```python
from build123d import *

# Parameters (mm, degrees)
F0_R          = 12.5
F1_DEPTH      = 20
F2_R          = 15
F3_DEPTH      = 4
F5_DEPTH      = 12
F7_DEPTH      = 7.4
F7_DEPTH_BACK = 5.4
F8_SIZE       = 0.5


with BuildPart() as f1:
    # F0 (on Top) → F1 (new body)
    with BuildSketch(Plane.XY):
        Circle(F0_R)
    extrude(amount=F1_DEPTH)

    # F2 (on face) → F3 (join)
    with BuildSketch(Plane.XY.offset(20)):
        Circle(F2_R)
    extrude(amount=F3_DEPTH)

    # F4 (on face) → F5 (join)
    with BuildSketch(Plane.XY.offset(24)):
        with BuildLine():
            ThreePointArc((-0.345779, 14.996014), (-2.25, 0), (-0.345779, -14.996014))
            ThreePointArc((-0.345779, -14.996014), (0, -15), (0.345779, -14.996014))
            ThreePointArc((0.345779, -14.996014), (2.25, 0), (0.345779, 14.996014))
            ThreePointArc((0.345779, 14.996014), (0, 15), (-0.345779, 14.996014))
        make_face()
    extrude(amount=F5_DEPTH)

    # F6 (on Right) → F7 (cut, two sides)
    with BuildSketch(Plane.YZ) as f7_sk:
        with BuildLine():
            Line((-12, 37), (-12, 36))
            ThreePointArc((-12, 36), (0, 30), (12, 36))
            Line((12, 36), (12, 37))
            Line((12, 37), (-12, 37))
        make_face()
    extrude(amount=F7_DEPTH, mode=Mode.SUBTRACT)
    extrude(f7_sk.sketch, amount=-F7_DEPTH_BACK, mode=Mode.SUBTRACT)

    # F8
    f8_edges = [f1.edges().sort_by_distance(p)[0] for p in [
        (-12.5, 0, 0),
        (-15, 0, 20),
    ]]
    chamfer(f8_edges, length=F8_SIZE)


solid = f1.part
```
Part model, mm, in its own coordinate system. A direction names the side the tool comes from. Round coordinates to 2 decimals unless told otherwise and drop trailing zeros. Write each loop counter-clockwise with the first axis right and the second up, starting at its lowest first coordinate (ties: lowest second). Pieces come first, ordered by that corner, then holes. Notation, with made-up numbers: (73.25, 21.5) -> (103.25, 21.5) arc R21 cw to (103.25, 60.5) -> close; hole circle Ø9 at (-3, 80). An arc over 180 degrees is marked (long way). Return JSON: item names as keys, results as strings. Group by question number.
Q1. Saw through at C-C on z = 2.5. Write the cut outline in (x, y).
Q2. Probe L1, parallel to Z at x = 7.5, y = -1.5; L2, parallel to Z at x = -12.75, y = -2.5; L3, parallel to Y at x = 8.25, z = 11. List the from-to ranges inside material, lowest first. Write a range as [from, to].
Q3. Pin check, flat tips, straight feed: pin 1 (8 mm diameter, centred on y = 9.5, z = 21.5, fed in from -X); pin 2 (1 mm diameter, centred on x = 8.5, y = -3.5, fed in from +Z); pin 3 (4 mm diameter, centred on y = 11.5, z = 27.5, fed in from +X). Stop position of each tip, or through.
Q4. Which spindle directions (+Z, -Z, +X, -X, +Y, -Y) get a long thin tool onto all of the face, cutting with end or side? Do faces 1 (the cylindrical face through (-2.25, 0.21, 28.58)), 2 (the cylindrical face through (2.25, -0.21, 28.58)), 3 (the cylindrical face through (11.923, 3.755, 10.114)). Say none if no direction does.
Q5. Saw through at B-B on z = 30.5. Write the cut outline in (x, y).
Q6. Saw through at A-A on y = 0. Write the cut outline in (x, z), plus the area to 4 significant figures.
Answer:
{
 "1": {"outline": "circle Ø25 at (0, 0)"},
 "2": {"L1": "[0, 24]", "L2": "[20, 24]", "L3": "[-9.39, 9.39]"},
 "3": {"pin 1": "x = -13.96", "pin 2": "z = 24", "pin 3": "x = 1.49"},
 "4": {"face 1": "+Z, -X", "face 2": "+Z, +X", "face 3": "-Z"},
 "5": {"outline": "(-2.13, -3.84) arc R60 ccw to (-0.35, -15) arc R15 ccw to (0.35, -15) arc R60 ccw to (2.13, -3.84) -> close; (-2.13, 3.84) -> (2.13, 3.84) arc R60 ccw to (0.35, 15) arc R15 ccw to (-0.35, 15) arc R60 ccw to start"},
 "6": {"outline": "(-15, 20.5) -> (-14.5, 20) -> (-12.5, 20) -> (-12.5, 0.5) -> (-12, 0) -> (12, 0) -> (12.5, 0.5) -> (12.5, 20) -> (14.5, 20) -> (15, 20.5) -> (15, 24) -> (2.25, 24) -> (2.25, 30) -> (-2.25, 30) -> (-2.25, 24) -> (-15, 24) -> close", "area": "646.5 mm2"}
}
